from build123d import *

# Parameters (mm, degrees)
BODY_S_W                    = 40
BODY_S_H                    = 26
BODY_S_R                    = 0.9
BODY_DEPTH                  = 2
CUTTING_S_R                 = 3.5
CUTTING_DEPTH               = 3
WING_S_W                    = 5
WING_S_H                    = 7
WING_S_R                    = 1.7
WING_DEPTH                  = 4
LINEARES_MUSTER2_COUNT      = 2
LINEARES_MUSTER2_PITCH      = 19
VERRUNDUNG2_R               = 2.5
GLIDES_S_W                  = 9.2
GLIDES_S_H                  = 26
GLIDES_DEPTH                = 0.7
GEAR_H_R                    = 7.5
GEARHOLE_DEPTH              = 1.5
SHAFT_BORE_DEPTH            = 29.460498942
SHAFT_BORE_DEPTH_BACK       = 29.460498942
BORE_S_R                    = 1.5
FASE2_SIZE                  = 3
FASE3_SIZE                  = 3
RAILCUT_W                   = 1.9
RAILCUT_H                   = 26
RAIL_CUT_DEPTH              = 1.8
EDGE_2_W                    = 0.3
EDGE_2_H                    = 26
CUT_EDGE_DEPTH              = 0.7
VERRUNDUNG6_R               = 0.6
VERRUNDUNG7_R               = 0.6
VERRUNDUNG8_R               = 0.6
GLIDE_SPACE_W               = 3
GLIDE_SPACE_H               = 26
GLIDE_SPACE_RACK_SPUR_DEPTH = 0.7
VERRUNDUNG10_R              = 0.5
VERRUNDUNG11_R              = 0.5
VERRUNDUNG12_R              = 0.5


# Some blends are built 0.0001 mm under size
with BuildPart() as part:
    # body-s → body (new, symmetric)
    with BuildSketch(Plane.XY):
        Rectangle(BODY_S_W, BODY_S_H)
        with Locations((-15, 8)):
            Circle(BODY_S_R, mode=Mode.SUBTRACT)
        with Locations((15, 8)):
            Circle(BODY_S_R, mode=Mode.SUBTRACT)
        with Locations((15, -8)):
            Circle(BODY_S_R, mode=Mode.SUBTRACT)
        with Locations((-15, -8)):
            Circle(BODY_S_R, mode=Mode.SUBTRACT)
        with Locations((0, -8)):
            Circle(BODY_S_R, mode=Mode.SUBTRACT)
    extrude(amount=BODY_DEPTH, both=True)

    # cutting-s → cutting (cut)
    with BuildSketch(Plane(origin=(0, 0, -2), x_dir=(-1, 0, 0), z_dir=(0, 0, -1))):
        with Locations((-15, 8)):
            Circle(CUTTING_S_R)
        with Locations((15, 8)):
            Circle(CUTTING_S_R)
        with Locations((15, -8)):
            Circle(CUTTING_S_R)
        with Locations((-15, -8)):
            Circle(CUTTING_S_R)
        with Locations((0, -8)):
            Circle(CUTTING_S_R)
    extrude(amount=-CUTTING_DEPTH, mode=Mode.SUBTRACT)

    # wing-s → wing (add)
    # profile 1 of 2: a face of its own
    with BuildSketch(Plane.XY.offset(2)):
        with Locations((-22.5, 9.5)):
            Rectangle(WING_S_W, WING_S_H)
        with Locations((-21.8, 9.5)):
            Circle(WING_S_R, mode=Mode.SUBTRACT)
    # profile 2 of 2: a face of its own
    with BuildSketch(Plane.XY.offset(2)):
        with Locations((22.5, 9.5)):
            Rectangle(WING_S_W, WING_S_H)
        with Locations((21.8, 9.5)):
            Circle(WING_S_R, mode=Mode.SUBTRACT)
    wing = extrude(amount=-WING_DEPTH)

    # Lineares Muster2: wing ×2
    with Locations(*[(0, -i * LINEARES_MUSTER2_PITCH, 0) for i in range(1, LINEARES_MUSTER2_COUNT)]):
        add(wing)

    # Verrundung2
    verrundung2_edges = [part.edges().sort_by_distance(p)[0] for p in [
        (25, -13, 0),
        (25, -6, 0),
        (-25, -6, 0),
        (-25, -13, 0),
        (-20, -6, 0),
        (-20, 6, 0),
        (-25, 6, 0),
        (-25, 13, 0),
        (25, 13, 0),
        (20, -6, 0),
        (20, 6, 0),
        (25, 6, 0),
    ]]
    fillet(verrundung2_edges, radius=VERRUNDUNG2_R - 0.0001)  # a hair under: the kernel refuses the full size

    # glides-s → glides (add)
    with BuildSketch(Plane.XY.offset(2)):
        with Locations((-8.1, 0)):
            Rectangle(GLIDES_S_W, GLIDES_S_H)
        with Locations((8.1, 0)):
            Rectangle(GLIDES_S_W, GLIDES_S_H)
    extrude(amount=GLIDES_DEPTH)

    # gear-h → gearhole (cut, symmetric)
    with BuildSketch(Plane.XY.offset(2)):
        with Locations(Location((0, 3.2, 0), (0, 0, 117.818139285))):
            Circle(GEAR_H_R)
    extrude(amount=GEARHOLE_DEPTH, both=True, mode=Mode.SUBTRACT)

    # bore-s → Shaft-bore (cut, two sides: drawn at the far end of the back side and taken through both)
    with BuildSketch(Plane.XY.offset(2).offset(-SHAFT_BORE_DEPTH_BACK)):
        with Locations((0, 3.2)):
            Circle(BORE_S_R)
    extrude(amount=SHAFT_BORE_DEPTH + SHAFT_BORE_DEPTH_BACK, mode=Mode.SUBTRACT)

    # Fase2
    # the kernel refuses this chamfer: 3 mm, written as the material it adds along each edge
    with BuildSketch(Plane(origin=(15, 8, 1), x_dir=(-1, 0, 0), z_dir=(0, -1, 0))) as fase2_piece_1_section:
        Polygon((3.5, FASE2_SIZE), (3.5 - FASE2_SIZE, 0), (3.5, 0), align=None)
    fase2_piece_1 = revolve(axis=Axis((15, 8, 1), (0, 0, -1)), mode=Mode.PRIVATE)
    fase2_piece_1 = split(fase2_piece_1, bisect_by=Plane(origin=(17.230122029, 8, -2), z_dir=(0, 0, 1)), keep=Keep.TOP, mode=Mode.PRIVATE)
    fase2_piece_1 = fase2_piece_1 - Plane(origin=(15, 8, -0.669877971), x_dir=(1, 0, 0), z_dir=(0, 0, -1)) * Cylinder(0.9, 14, mode=Mode.PRIVATE)
    add(fase2_piece_1)

    # Fase3
    # the kernel refuses this chamfer: 3 mm, written as the material it adds along each edge
    with BuildSketch(Plane(origin=(-15, -8, 1), x_dir=(-1, 0, 0), z_dir=(0, -1, 0))) as fase3_piece_1_section:
        Polygon((3.5, FASE3_SIZE), (3.5 - FASE3_SIZE, 0), (3.5, 0), align=None)
    fase3_piece_1 = revolve(axis=Axis((-15, -8, 1), (0, 0, -1)), mode=Mode.PRIVATE)
    fase3_piece_1 = split(fase3_piece_1, bisect_by=Plane(origin=(-12.769877971, -8, -2), z_dir=(0, 0, 1)), keep=Keep.TOP, mode=Mode.PRIVATE)
    fase3_piece_1 = fase3_piece_1 - Plane(origin=(-15, -8, -0.669877971), x_dir=(1, 0, 0), z_dir=(0, 0, -1)) * Cylinder(0.9, 14, mode=Mode.PRIVATE)
    add(fase3_piece_1)
    with BuildSketch(Plane(origin=(-15, 8, 1), x_dir=(-1, 0, 0), z_dir=(0, -1, 0))) as fase3_piece_2_section:
        Polygon((3.5, FASE3_SIZE), (3.5 - FASE3_SIZE, 0), (3.5, 0), align=None)
    fase3_piece_2 = revolve(axis=Axis((-15, 8, 1), (0, 0, -1)), mode=Mode.PRIVATE)
    fase3_piece_2 = split(fase3_piece_2, bisect_by=Plane(origin=(-12.769877971, 8, -2), z_dir=(0, 0, 1)), keep=Keep.TOP, mode=Mode.PRIVATE)
    fase3_piece_2 = fase3_piece_2 - Plane(origin=(-15, 8, -0.669877971), x_dir=(1, 0, 0), z_dir=(0, 0, -1)) * Cylinder(0.9, 14, mode=Mode.PRIVATE)
    add(fase3_piece_2)
    with BuildSketch(Plane(origin=(0, -8, 1), x_dir=(-1, 0, 0), z_dir=(0, -1, 0))) as fase3_piece_3_section:
        Polygon((3.5, FASE3_SIZE), (3.5 - FASE3_SIZE, 0), (3.5, 0), align=None)
    fase3_piece_3 = revolve(axis=Axis((0, -8, 1), (0, 0, -1)), mode=Mode.PRIVATE)
    fase3_piece_3 = split(fase3_piece_3, bisect_by=Plane(origin=(2.230122029, -8, -2), z_dir=(0, 0, 1)), keep=Keep.TOP, mode=Mode.PRIVATE)
    fase3_piece_3 = fase3_piece_3 - Plane(origin=(0, -8, -0.669877971), x_dir=(1, 0, 0), z_dir=(0, 0, -1)) * Cylinder(0.9, 14, mode=Mode.PRIVATE)
    add(fase3_piece_3)
    with BuildSketch(Plane(origin=(15, -8, 1), x_dir=(-1, 0, 0), z_dir=(0, -1, 0))) as fase3_piece_4_section:
        Polygon((3.5, FASE3_SIZE), (3.5 - FASE3_SIZE, 0), (3.5, 0), align=None)
    fase3_piece_4 = revolve(axis=Axis((15, -8, 1), (0, 0, -1)), mode=Mode.PRIVATE)
    fase3_piece_4 = split(fase3_piece_4, bisect_by=Plane(origin=(17.230122029, -8, -2), z_dir=(0, 0, 1)), keep=Keep.TOP, mode=Mode.PRIVATE)
    fase3_piece_4 = fase3_piece_4 - Plane(origin=(15, -8, -0.669877971), x_dir=(1, 0, 0), z_dir=(0, 0, -1)) * Cylinder(0.9, 14, mode=Mode.PRIVATE)
    add(fase3_piece_4)

    # railcut → rail-cut (cut)
    with BuildSketch(Plane.XY.offset(2.7)):
        with Locations((-11.45, 0)):
            Rectangle(RAILCUT_W, RAILCUT_H)
        with Locations((11.45, 0)):
            Rectangle(RAILCUT_W, RAILCUT_H)
    extrude(amount=-RAIL_CUT_DEPTH, mode=Mode.SUBTRACT)

    # edge 2 → cut-edge (cut)
    with BuildSketch(Plane.XY.offset(2.7)):
        with Locations((-12.55, 0)):
            Rectangle(EDGE_2_W, EDGE_2_H)
        with Locations((12.55, 0)):
            Rectangle(EDGE_2_W, EDGE_2_H)
    extrude(amount=-CUT_EDGE_DEPTH, mode=Mode.SUBTRACT)

    # Verrundung6
    verrundung6_edges = [part.edges().sort_by_distance(p)[0] for p in [
        (-12.4, 0, 2),
        (12.4, 0, 2),
    ]]
    fillet(verrundung6_edges, radius=VERRUNDUNG6_R)

    # Verrundung7
    verrundung7_edges = [part.edges().sort_by_distance(p)[0] for p in [
        (12.4, 0, 0.9),
        (10.5, 0, 0.9),
        (-12.4, 0, 0.9),
        (-10.5, 0, 0.9),
    ]]
    fillet(verrundung7_edges, radius=VERRUNDUNG7_R)

    # Verrundung8
    verrundung8_edges = [part.edges().sort_by_distance(p)[0] for p in [
        (-10.5, 0, 2.7),
        (10.5, 0, 2.7),
    ]]
    fillet(verrundung8_edges, radius=VERRUNDUNG8_R)

    # glide-space → glide-space-rack-spur (cut)
    with BuildSketch(Plane.XY.offset(2.7)):
        with Locations((-5, 0)):
            Rectangle(GLIDE_SPACE_W, GLIDE_SPACE_H)
        with Locations((5, 0)):
            Rectangle(GLIDE_SPACE_W, GLIDE_SPACE_H)
    extrude(amount=-GLIDE_SPACE_RACK_SPUR_DEPTH, mode=Mode.SUBTRACT)

    # Verrundung10
    verrundung10_edges = [part.edges().sort_by_distance(p)[0] for p in [
        (-6.5, 9.970828693, 2.7),
    ]]
    fillet(verrundung10_edges, radius=VERRUNDUNG10_R)

    # Verrundung11
    verrundung11_edges = [part.edges().sort_by_distance(p)[0] for p in [
        (-6.5, -6.770828693, 2.7),
    ]]
    fillet(verrundung11_edges, radius=VERRUNDUNG11_R)

    # Verrundung12
    verrundung12_edges = [part.edges().sort_by_distance(p)[0] for p in [
        (6.5, 9.970828693, 2.7),
        (6.5, -6.770828693, 2.7),
    ]]
    fillet(verrundung12_edges, radius=VERRUNDUNG12_R)


solid = part.part
Verification items for the finished model (mm, model axes). A direction names the side the tool comes from. Round coordinates to 2 decimals unless told otherwise and drop trailing zeros. Order: outer loops, then holes, each group sorted by start corner. A loop starts at its lowest first (then second) coordinate and runs counter-clockwise, first axis right, second up. Notation, with made-up numbers: (23.25, -7.75) -> (56.25, -7.75) arc R20 ccw to (56.25, 5.25) -> close; hole circle Ø1 at (23.5, 73). An arc over 180 degrees is marked (long way). Put each result on its own line as item: value.
1) Section check D-D (x = 15). Record the cut outline in (y, z).
Final values:
outline: (-13, -2) -> (-11.5, -2) -> (-8.9, 0.6) -> (-8.9, 2) -> (-13, 2) -> close; (-7.1, 0.6) -> (-4.5, -2) -> (4.5, -2) -> (7.1, 0.6) -> (7.1, 2) -> (-7.1, 2) -> close; (8.9, 0.6) -> (11.5, -2) -> (13, -2) -> (13, 2) -> (8.9, 2) -> close
2) Section check A-A (z = -0.5). Give the number of separate pieces and of enclosed holes in the cut face, then the cut area to 3 significant figures.
Final values:
separate pieces: 1
enclosed holes: 10
area: 1,070 mm^2
3) Section check B-B (x = 0). Record the cut outline in (y, z), then the cut area to 3 significant figures.
Final values:
outline: (-13, -2) -> (-11.5, -2) -> (-8.9, 0.6) -> (-8.9, 2) -> (-13, 2) -> close; (-7.1, 0.6) -> (-4.5, -2) -> (1.7, -2) -> (1.7, 0.5) -> (-4.3, 0.5) -> (-4.3, 2) -> (-7.1, 2) -> close; (4.7, -2) -> (13, -2) -> (13, 2) -> (10.7, 2) -> (10.7, 0.5) -> (4.7, 0.5) -> close
area: 60.0 mm^2
4) Section check C-C (x = -21). Record the cut outline in (y, z), then the cut area to 3 significant figures.
Final values:
outline: (-13, -2) -> (-11, -2) -> (-11, 2) -> (-13, 2) -> close; (-8, -2) -> (-5.5, -2) -> (-5.5, 2) -> (-8, 2) -> close; (5.5, -2) -> (8, -2) -> (8, 2) -> (5.5, 2) -> close; (11, -2) -> (13, -2) -> (13, 2) -> (11, 2) -> close
area: 36.0 mm^2
5) Set-up check for faces 5 (the flat face through (-0.1, -9.5, 2)), 6 (the cylindrical face through (20.713, -5.248, -0.028)), 7 (the flat face through (-18, 0, 2)): record each of +Z, -Z, +X, -X, +Y, -Y from which the full face is reachable in a straight line by a thin tool's end or side.
Final values:
face 5: +Z, +Y, -Y
face 6: +Z, -Z, +X
face 7: +Z, -X, +Y, -Y
6) Mould release check, pull along Y, two halves, no side actions. Record for faces 1 (the cylindrical face through (-24.287, -12.248, -0.028)), 2 (the flat face through (25, -10, 0)), 3 (the flat face through (20, 0, 0)), 4 (the cylindrical face through (24.248, 12.287, -0.028)): +Y half, -Y half, draft (parallel to the pull), parting line (faces both ways), or undercut.
Final values:
face 1: -Y half
face 2: draft
face 3: undercut
face 4: +Y half
7) Depth check by flat-ended pin: pin 1 (1.8 mm diameter, centred on x = 1.5, y = 10.5, fed in from +Z); pin 2 (0.8 mm diameter, centred on x = 11.5, y = 0, fed in from +Z); pin 3 (0.5 mm diameter, centred on y = 3.5, z = 2, fed in from -X). Enter the tip coordinate at first touch or a pass-through.
Final values:
pin 1: stops at z = 2
pin 2: stops at z = 0.91
pin 3: stops at x = -20.01
8) Material ranges on line 1 (X direction, y = -8.5, z = 0.85); line 2 (Y direction, x = -21.8, z = -0.2); line 3 (Y direction, x = 0, z = 1), recorded low to high.
Final values:
line 1: x = -25 to -23.17, -20.43 to -15.75, -14.25 to -0.75, 0.75 to 14.25, 15.75 to 20.43, 23.17 to 25
line 2: y = -13 to -11.2, -7.8 to -5.9, 5.9 to 7.8, 11.2 to 13
line 3: y = -13 to -8.9, -7.1 to -4.3, 10.7 to 13
